Read the model definition and answer for the solid it produces. Units are mm, in the model's axes. Coordinates: 2 decimals unless noted, no trailing zeros. Loops run counter-clockwise (first coordinate to the right, second up) from the corner with the lowest first, then second, coordinate; pieces in that order, holes last. Notation, with made-up numbers: (-28.5, 33) - (12.5, 33) arc R19 ccw to (12.5, 64) - close; hole circle Ø5 at (17.5, 13). An arc over 180 degrees is marked (long way). Use one line per item in the form item = value. Start each with the question number.
1) A cutting plane is placed at A-A (x = 0). Give the vertices of the cut face in (y, z).
2) A cutting plane is placed at D-D (y = 16.5). Give the vertices of the cut face in (x, z).
3) A cutting plane is placed at C-C (y = 168.5). Give the vertices of the cut face in (x, z), and give its area (3 significant figures).
4) Each of these flat-tipped pins is pushed along its axis until it touches: P1, Ø1.5, axis at y = 203.5, z = 0, coming from the -X side; P2, Ø1, axis at y = 88.5, z = -0.5, coming from the -X side; P3, Ø6.5, axis at x = 0, y = 16.5, coming from the +Z side; P4, Ø0.9, axis at y = 201.5, z = 0.5, coming from the -X side. Where does it stop, or does it pass through?
5) Consider line 1 (X direction, y = 202.5, z = 0.4); line 2 (X direction, y = 201, z = -0.65); line 3 (X direction, y = 60, z = 1.25). Determine where each line is inside the solid, lowest interval first.
6) A cutting plane is placed at B-B (z = 0.6). Give the vertices of the cut face in (x, y).
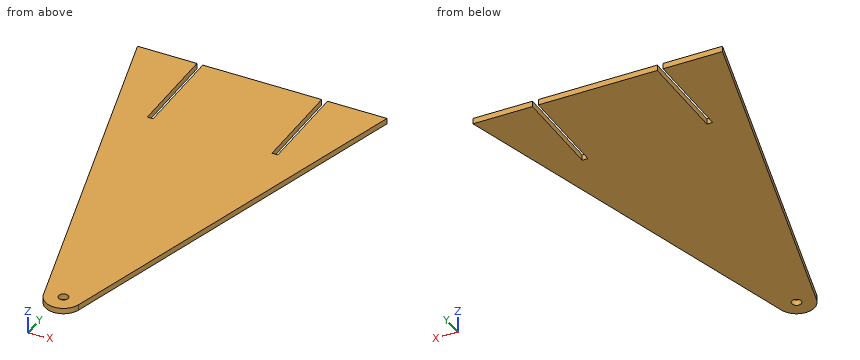
Autodesk Inventor part; units mm, degrees
ref_plane "YZ Plane" through (0, 0, 0) normal (1, 0, 0) x (0, 1, 0)
ref_plane "XZ Plane" through (0, 0, 0) normal (0, 1, 0) x (-1, 0, 0)
ref_plane "XY Plane" through (0, 0, 0) normal (0, 0, 1) x (1, 0, 0)
sketch "Sketch1" plane through (0, 0, 0) normal (0, 0, 1) x (1, 0, 0)
  circle A0 centre (0, 16.5) radius 2.5
  line L0 (0, 16.5) -> (0, 216.5) construction
  arc A1 (-9.1582, 13.9748) -> (9.1582, 13.9748) centre (0, 16.5) ccw
  line L1 (65, 216.5) -> (9.1582, 13.9748)
  circle A2 centre (0, 16.5) radius 2.5
  line L2 (34, 216.5) -> (34, 166.5)
  line L3 (34, 166.5) -> (31, 166.5)
  line L4 (31, 166.5) -> (31, 216.5)
  line L5 (0, 216.5) -> (31, 216.5)
  line L6 (34, 216.5) -> (65, 216.5)
  line L7 (-65, 216.5) -> (-9.1582, 13.9748)
  line L8 (-34, 216.5) -> (-34, 166.5)
  line L9 (-34, 166.5) -> (-31, 166.5)
  line L10 (-31, 166.5) -> (-31, 216.5)
  line L11 (0, 216.5) -> (-31, 216.5)
  line L12 (-34, 216.5) -> (-65, 216.5)
  point P0 (0, 0)
  dimension "d0" = 200
  dimension "d1" = 65
  dimension "d2" = 19
  dimension "d7" = 50
  dimension "d8" = 3
  dimension "d9" = 31
extrude "Extrusion2" add sketch "Sketch1" along normal blind 1.5 and the other way blind 1.5
properties part number "Pivote_Estructura"
Found:
q1.outline = (7, -1.5) - (14, -1.5) - (14, 1.5) - (7, 1.5) - close; (19, -1.5) - (216.5, -1.5) - (216.5, 1.5) - (19, 1.5) - close
q2.outline = (-9.85, -1.5) - (-2.5, -1.5) - (-2.5, 1.5) - (-9.85, 1.5) - close; (2.5, -1.5) - (9.85, -1.5) - (9.85, 1.5) - (2.5, 1.5) - close
q3.outline = (-51.77, -1.5) - (-34, -1.5) - (-34, 1.5) - (-51.77, 1.5) - close; (-31, -1.5) - (31, -1.5) - (31, 1.5) - (-31, 1.5) - close; (34, -1.5) - (51.77, -1.5) - (51.77, 1.5) - (34, 1.5) - close
q3.area = 293 mm^2
q4.P1 = -61.62
q4.P2 = -29.84
q4.P3 = 1.5
q4.P4 = -60.99
q5.line_1 = -61.14 to -34, -31 to 31, 34 to 61.14
q5.line_2 = -60.73 to -34, -31 to 31, 34 to 60.73
q5.line_3 = -21.85 to 21.85
q6.outline = (-65, 216.5) - (-9.16, 13.97) arc R9.5 ccw to (9.16, 13.97) - (65, 216.5) - (34, 216.5) - (34, 166.5) - (31, 166.5) - (31, 216.5) - (-31, 216.5) - (-31, 166.5) - (-34, 166.5) - (-34, 216.5) - close; hole circle Ø5 at (0, 16.5)
